Check sheet for the modelled part. Datum: model origin and axes. Units: mm. Give positions to 0.01 mm unless a question says otherwise; leave off trailing zeros. Order: outer loops, then holes, each group sorted by start corner. A loop starts at its lowest first (then second) coordinate and runs counter-clockwise, first axis right, second up.
Item 1: Sectioned sample at A-A on z = 3.25. Record the boundary of the cut face in (x, y).
Item 2: Sectioned sample at B-B on y = 4.75. Record the boundary of the cut face in (x, z), and give its area (3 significant figures).
Item 3: Sectioned sample at C-C on x = 0. Record the boundary of the cut face in (y, z), and give its area (3 significant figures).
Item 4: Release check for a two-part mould opening along Y. For faces 1 (the flat face through (-4.12, 4.4, 7.14)), 2 (the cylindrical face through (-10.89, -1.06, 5.04)), 3 (the cylindrical face through (-11.11, -8.52, 3.98)), 4 (the cylindrical face through (-1.39, 6.94, 3.92)) record: released by +Y, released by -Y, zero draft, split by the parting line, or undercut.
Item 5: Material ranges on line 1 along X through (y, z) = (0, 4.25); line 2 along Y through (x, z) = (0, 5.25); line 3 along X through (y, z) = (0, 7.25), recorded low to high.
Item 6: Gauge pin test, flat ends, axial feed: P1, Ø4, axis at x = -9.5, y = 0, coming from the +Z side; P2, Ø5.5, axis at x = 9.5, y = 0, coming from the -Z side; P3, Ø5, axis at y = 5, z = 8.5, coming from the -X side (3 decimals); P4, Ø6, axis at x = 0, y = 0, coming from the +Z side. Record the tip position at first contact, or that the pin passes through.
Item 7: Sectioned sample at D-D on y = 1.25. Record the boundary of the cut face in (x, z), and give its area (3 significant figures).
from build123d import *

# Parameters (mm, degrees)
F0_R     = 14
F0_R_2   = 1.75
F0_R_3   = 5.1
F1_DEPTH = 10
F6_DEPTH = 40


with BuildPart() as f1:
    # F0 (on Top) → F1 (new body)
    with BuildSketch(Plane.XY):
        Circle(F0_R)
        with Locations((0, -8)):
            Circle(F0_R_2, mode=Mode.SUBTRACT)
        with Locations((-9.5, 0)):
            Circle(F0_R_2, mode=Mode.SUBTRACT)
        Circle(F0_R_3, mode=Mode.SUBTRACT)
        with Locations((9.5, 0)):
            Circle(F0_R_2, mode=Mode.SUBTRACT)
        with Locations((0, 8)):
            Circle(F0_R_2, mode=Mode.SUBTRACT)
    extrude(amount=F1_DEPTH)

    # F5 (on face) → F6 (intersect)
    with BuildSketch(Plane(origin=(17.6564226245, -17.6564226245, -1.2253490154), x_dir=(0.7045622489, 0.7079556371, -0.0488963521), z_dir=(0.706256905, -0.706256905, -0.0490139606))):
        Polygon((-42.1593469174, 12.1424701935), (-41.5246425416, -0.8069908946), (14.9219552549, 1.9596804268), (14.7750896798, 4.9560833541), align=None)
        Polygon((14.7750896798, 4.9560833541), (14.9219552549, 1.9596804268), (31.9154007009, 2.7925964926), align=None)
    extrude(amount=-F6_DEPTH, mode=Mode.INTERSECT)


solid = f1.part
Report:
1. outline: circle Ø28 at (0, 0); hole circle Ø3.5 at (-9.5, 0); hole circle Ø10.2 at (0, 0); hole circle Ø3.5 at (0, -8); hole circle Ø3.5 at (0, 8); hole circle Ø3.5 at (9.5, 0)
2. outline: (-13.17, 1.85) - (-1.86, 1.46) - (-1.86, 6.75) - (-13.17, 8.55) - close; (1.86, 1.33) - (13.17, 0.94) - (13.17, 4.35) - (1.86, 6.16) - close
2. area: 114 mm2
3. outline: (-14, 0.74) - (-9.75, 0.89) - (-9.75, 7.76) - (-14, 8.14) - close; (-6.25, 1.01) - (-5.1, 1.05) - (-5.1, 7.34) - (-6.25, 7.44) - close; (5.1, 1.41) - (6.25, 1.45) - (6.25, 6.32) - (5.1, 6.42) - close; (9.75, 1.57) - (14, 1.71) - (14, 5.62) - (9.75, 6) - close
3. area: 61.0 mm2
4. face 1: released by +Y
4. face 2: undercut
4. face 3: split by the parting line
4. face 4: undercut
5. line 1: x = -14 to -11.25, -7.75 to -5.1, 5.1 to 7.75, 11.25 to 14
5. line 2: y = -14 to -9.75, -6.25 to -5.1, 5.1 to 6.25, 9.75 to 14
5. line 3: x = -14 to -11.25, -7.75 to -5.1
6. P1: stops at z = 8.76
6. P2: stops at z = 0.76
6. P3: stops at x = -13.775
6. P4: passes through
7. outline: (-13.94, 1.76) - (-10.72, 1.64) - (-10.72, 8.48) - (-13.94, 8.99) - close; (-8.28, 1.56) - (-4.94, 1.44) - (-4.94, 7.56) - (-8.28, 8.09) - close; (4.94, 1.1) - (8.28, 0.98) - (8.28, 5.45) - (4.94, 5.98) - close; (10.72, 0.9) - (13.94, 0.79) - (13.94, 4.54) - (10.72, 5.06) - close
7. area: 72.0 mm2
